from build123d import *

# Parameters (mm, degrees)
F2_DEPTH = 1.625
F3_R     = 0.5


with BuildPart() as f2:
    # F1 (on Front) → F2 (new body, symmetric)
    with BuildSketch(Plane.XZ):
        with BuildLine():
            ThreePointArc((0, -6.875), (-2.0724417463, -6.5551971906), (-3.9520768911, -5.6255411515))
            ThreePointArc((-3.9520768911, -5.6255411515), (-4.8570002775, -7.1160909953), (-6.5757097792, -6.8217054979))
            ThreePointArc((-6.5757097792, -6.8217054979), (-7.4894639741, -8.9857797177), (-9.0066893746, -10.7791539234))
            ThreePointArc((-9.0066893746, -10.7791539234), (-10.3561219729, -10.7473840389), (-10.4445927673, -9.400479966))
            ThreePointArc((-10.4445927673, -9.400479966), (-8.8177667586, -7.5260240462), (-7.0479231089, -5.7859661986))
            ThreePointArc((-7.0479231089, -5.7859661986), (-6.6159518229, -4.6300438958), (-5.4766665535, -4.1559293139))
            ThreePointArc((-5.4766665535, -4.1559293139), (-6.1554446566, -3.3057655277), (-6.7033968415, -2.3659428957))
            ThreePointArc((-6.7033968415, -2.3659428957), (-7.5646836603, -2.8179203379), (-8.2709699391, -3.4866940551))
            Line((-8.2709699391, -3.4866940551), (-12.0057025921, -8.1503055323))
            ThreePointArc((-12.0057025921, -8.1503055323), (-11.8324993376, -12.098674705), (-7.8959026306, -12.4491384793))
            ThreePointArc((-7.8959026306, -12.4491384793), (-4.1524531082, -10.534781214), (0, -9.875))
            Line((0, -9.875), (0, -6.875))
        make_face()
    extrude(amount=F2_DEPTH, both=True)

    # F3
    f3_edges = [f2.edges().sort_by_distance(p)[0] for p in [
        (-3.952077, 0, -5.625541),
        (-7.047923, 0, -5.785966),
        (-6.703397, 0, -2.365943),
        (-5.476667, 0, -4.155929),
        (-6.57571, 0, -6.821705),
    ]]
    fillet(f3_edges, radius=F3_R)

    # F4: F2 across plane


with BuildPart() as f2_1:
    add(f2.part)
    add(f2.part.mirror(Plane.YZ))


solid = f2_1.part
CAD build for the part. Positions are in the model's coordinates, mm. A direction names the side the tool comes from. Coordinates: 2 decimals unless noted, no trailing zeros. Write each loop counter-clockwise with the first axis right and the second up, starting at its lowest first coordinate (ties: lowest second). Pieces come first, ordered by that corner, then holes. Notation, with made-up numbers: (9.25, 15.5) - (31.25, 15.5) arc R21 cw to (31.25, 32.5) - close; hole circle Ø9 at (-14, 15). An arc over 180 degrees is marked (long way). Use a Markdown table: item, result. Add a question column.
Item 1: 3-axis set-ups, long thin cutter, end or side, ignore diameter. For faces 1 (the face through (0, -1.625, -9)), 2 (the face through (-6.787, -0.023, -4.841)): which of +Z, -Z, +X, -X, +Y, -Y reach the whole face in a straight line?
Item 2: Band-saw the part on C-C, the plane z = -8.75. Give the cut face in (x, y) (3 decimals), and give its area (3 significant figures).
Item 3: Mould opens along X. For faces 3 (the face through (7.8, 0, -3)), 4 (the face through (0, 1.625, -9)), 5 (the face through (-10.34, -0.02, -10.76)), 6 (the face through (7.647, -0.023, -9.232)) say: pulls with the +X half, pulls with the -X half, needs draft (parallel to the pull), parting line crosses it, or undercut.
Item 4: Band-saw the part on D-D, the plane z = -11.5. Give the cut face in (x, y) (3 decimals).
Item 5: Band-saw the part on B-B, the plane x = 7.5. Give the cut face in (y, z) (3 decimals).
Item 6: Band-saw the part on A-A, the plane z = -6.5. Give the cut face in (x, y) (3 decimals), and give its area (3 significant figures).
Item 7: Drill centre lines: L1, parallel to X at y = 1.25, z = -8.75; L2, parallel to X at y = 0.45, z = -8; L3, parallel to Z at x = 8.25, y = -0.55. Where is each one in solid material? Low to high. Write a range as from..to.
Numbers:
| question | item | result |
|---|---|---|
| 1 | face 1 | +Z, -Z, +X, -X, -Y |
| 1 | face 2 | +Y, -Y |
| 2 | outline | (-12.379, -1.625) - (-9.909, -1.625) - (-9.909, 1.625) - (-12.379, 1.625) - close; (-7.35, -1.625) - (7.35, -1.625) - (7.35, 1.625) - (-7.35, 1.625) - close; (9.909, -1.625) - (12.379, -1.625) - (12.379, 1.625) - (9.909, 1.625) - close |
| 2 | area | 63.8 mm2 |
| 3 | face 3 | pulls with the +X half |
| 3 | face 4 | needs draft |
| 3 | face 5 | undercut |
| 3 | face 6 | undercut |
| 4 | outline | (-12.277, -1.625) - (-6.395, -1.625) - (-6.395, 1.625) - (-12.277, 1.625) - close; (6.395, -1.625) - (12.277, -1.625) - (12.277, 1.625) - (6.395, 1.625) - close |
| 5 | outline | (-1.625, -12.171) - (1.625, -12.171) - (1.625, -9.003) - (-1.625, -9.003) - close; (-1.625, -6.205) - (1.625, -6.205) - (1.625, -2.773) - (-1.625, -2.773) - close |
| 6 | outline | (-10.684, -1.625) - (-7.808, -1.625) - (-7.808, 1.625) - (-10.684, 1.625) - close; (-4.169, -1.625) - (-2.24, -1.625) - (-2.24, 1.625) - (-4.169, 1.625) - close; (2.24, -1.625) - (4.169, -1.625) - (4.169, 1.625) - (2.24, 1.625) - close; (7.808, -1.625) - (10.684, -1.625) - (10.684, 1.625) - (7.808, 1.625) - close |
| 6 | area | 31.2 mm2 |
| 7 | L1 | -12.38..-9.91, -7.35..7.35, 9.91..12.38 |
| 7 | L2 | -11.89..-9.25, -6.98..6.98, 9.25..11.89 |
| 7 | L3 | -12.67..-10.02, -6.94..-3.46 |
